Geometry: see drawing. Coordinates: mm, zero at the bounding-box minimum. Give positions to 0.01 mm unless a question says otherwise; leave off trailing zeros. Loops run counter-clockwise (first coordinate to the right, second up) from the corner with the lowest first, then second, coordinate; pieces in that order, holes last. Notation, with made-up numbers: (86, 86.5) -> (100, 86.5) arc R14 ccw to (100, 94.5) -> close; hole circle Ø4 at (7, 65.5). An arc over 180 degrees is marked (long way). Answer in a Markdown table with one row per item. Add a question column.
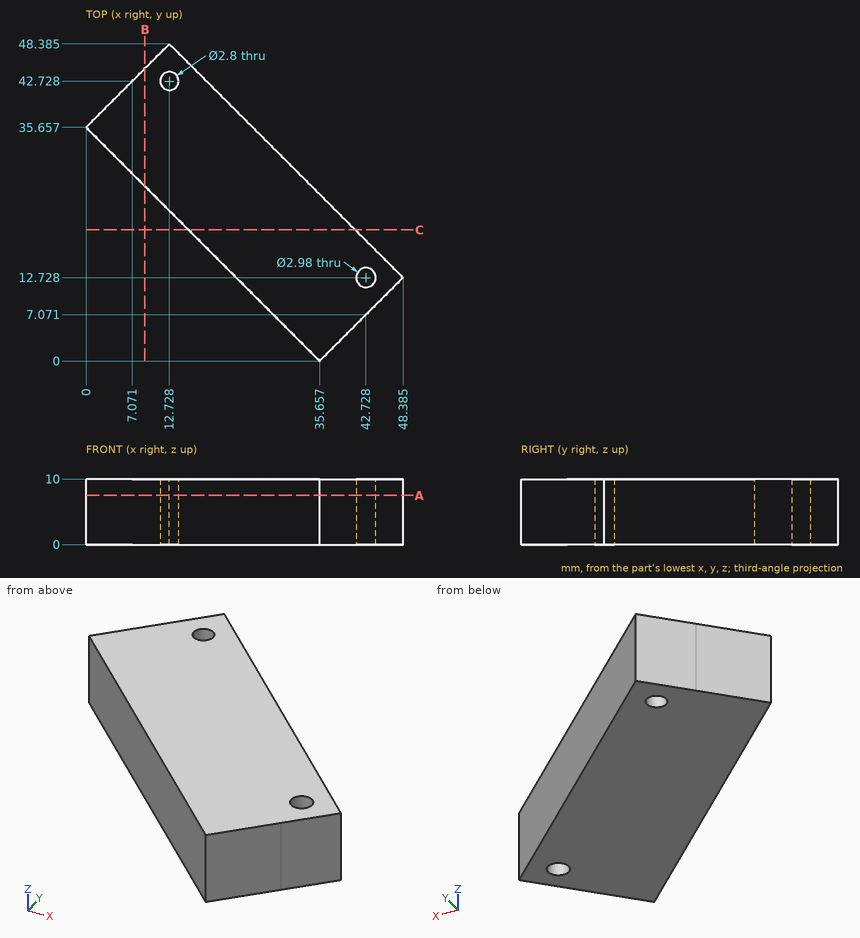
1) Section A-A on z = 7.5. Output: boundary loops of the cut face in (x, y) (1 decimal).
2) Section B-B on x = 9. Output: boundary loops of the cut face in (y, z).
3) Section C-C on y = 20. Output: boundary loops of the cut face in (x, z), and give its area (3 significant figures).
4) Material intervals for line 1 along Y through (x, z) = (14, 7.5) (1 decimal); line 2 along Y through (x, z) = (13.5, 9.5) (1 decimal); line 3 along X through (y, z) = (35, 5), sorted ascending.
5) Pin query (flat end, axial travel): pin 1 (3 mm diameter, centred on y = 18, z = 3.5, fed in from -X); pin 2 (5 mm diameter, centred on x = 32, z = 5, fed in from +Y); pin 3 (1.5 mm diameter, centred on y = 27.5, z = 8, fed in from +X). Return the tip coordinate at first contact, or that it passes through.
Working result:
| question | item | result |
|---|---|---|
| 1 | outline | (0, 35.7) -> (35.7, 0) -> (42.7, 7.1) -> (48.4, 12.7) -> (12.7, 48.4) -> (7.1, 42.7) -> close; hole circle Ø2.8 at (12.7, 42.7); hole circle Ø3 at (42.7, 12.7) |
| 2 | outline | (26.66, 0) -> (44.66, 0) -> (44.66, 10) -> (26.66, 10) -> close |
| 3 | outline | (15.66, 0) -> (41.11, 0) -> (41.11, 10) -> (15.66, 10) -> close |
| 3 | area | 255 mm2 |
| 4 | line 1 | y = 21.7 to 42.1, 43.3 to 47.1 |
| 4 | line 2 | y = 22.2 to 41.6, 43.9 to 47.6 |
| 4 | line 3 | x = 0.66 to 26.11 |
| 5 | pin 1 | stops at x = 16.16 |
| 5 | pin 2 | stops at y = 31.61 |
| 5 | pin 3 | stops at x = 34.36 |
